Design review of the part built by this model. Coordinates are the model's own, in mm. A direction names the side the tool comes from. Round coordinates to 2 decimals unless told otherwise and drop trailing zeros. Write each loop counter-clockwise with the first axis right and the second up, starting at its lowest first coordinate (ties: lowest second). Pieces come first, ordered by that corner, then holes. Notation, with made-up numbers: (-4.75, -14) -> (46.25, -14) arc R22 ccw to (46.25, -2) -> close; hole circle Ø10 at (56, 24.5). An arc over 180 degrees is marked (long way). One line per question, with ' | ' between items. Start each with the question number.
1) Mouldability with a two-part tool opening along Z and no side actions: class faces 1 (the cylindrical face through (-85.51, 20.27, 4.03)), 2 (the cylindrical face through (-13.046, 7.296, 5.042)), 3 (the flat face through (-23, 4, 6)), 4 (the flat face through (-46, 79, 2)) as +Z half, -Z half, draft (parallel to the pull), parting line (faces both ways), or undercut.
2) For faces 5 (the flat face through (-6, 23, 5)), 6 (the flat face through (-67, 152, 6)), 7 (the cylindrical face through (-4.296, 10.389, 5.042)), 8 (the cylindrical face through (-8.31, 12.01, 5.04)), 9 (the flat face through (-85, 137, 6)), list the 3-axis set-ups (+Z, -Z, +X, -X, +Y, -Y) from which the entire face can be reached by the end or side of a thin tool; tool diameter is ignored.
3) Insertion check: pin 1 Ø1 at (y, z) = (19.5, 4.5) entering from +X; pin 2 Ø3 at (x, z) = (-35.5, 5.5) entering from -Y; pin 3 Ø10 at (x, y) = (-13.5, 95.5) entering from +Z. Each pin has a flat end and moves straight along its axis. Give the tip position at first contact, or say it passes through.
4) For probe 1 along Y at (x, z) = (-43, 6); probe 2 along X at (y, z) = (3.6, 5); probe 3 along Z at (x, y) = (-67, 151.3), list the stretches that pass through material, from the lowest coordinate up.
5) Consider section A-A (x = -39.5). Give the boundary of the cut face in (y, z), then the cut area to 3 significant figures.
6) Consider section B-B (y = 102.5). Give the boundary of the cut face in (x, z).
```python
from build123d import *

# Parameters (mm, degrees)
SKETCH_1_W                = 90
SKETCH_1_H                = 156
EXTRUDE_1_DEPTH           = 2
CHAMFER_1_SIZE            = 10
FILLET_648_R              = 2
EXTRUDE_2_DEPTH           = 6
SHELL_3_T                 = -4
SHELL_3_THICKNESS_2_DEPTH = 2
SKETCH_17_W               = 18.399609766
SKETCH_17_H               = 163.649147631
SKETCH_17_W_2             = 16.459731854
SKETCH_17_H_2             = 168.058563627
CUT_EXTRUDE_14_DEPTH      = 6
SKETCH_8_W                = 109.527726605
SKETCH_8_H                = 110
CUT_EXTRUDE_4177_DEPTH    = 6
EXTRUDE_5_DEPTH           = 6
SKETCH_5_R                = 0.8
CUT_EXTRUDE_5486_DEPTH    = 200
FILLET_5638_R             = 4
SKETCH_4_R                = 0.8
CUT_EXTRUDE_6124_DEPTH    = 100
SKETCH_6_W                = 5
SKETCH_6_H                = 14
EXTRUDE_C_DEPTH           = 6
SKETCH_9_R                = 0.8
CUT_EXTRUDE_C_DEPTH       = 50
SKETCH_23_R               = 1.6
CUT_EXTRUDE_16_DEPTH      = 1
CUT_EXTRUDE_START         = -1
SKETCH_24_R               = 1.6
CUT_EXTRUDE_17_DEPTH      = 1
SKETCH_22_R               = 1.6
CUT_EXTRUDE_15_DEPTH      = 1
SKETCH_13_R               = 1.6
CUT_EXTRUDE_10_DEPTH      = 1
SKETCH_18_W               = 2
SKETCH_18_H               = 96
EXTRUDE_4_DEPTH           = 6
FILLET_1_R                = 4
FILLET_2_R                = 0.5
SKETCH_25_W               = 24.531639896
SKETCH_25_H               = 27.877987264
CUT_EXTRUDE_18_DEPTH      = 10


with BuildPart() as part:
    # 草图1 → 凸台-拉伸1 (new body)
    with BuildSketch(Plane.XY):
        with Locations((-45, 78)):
            Rectangle(SKETCH_1_W, SKETCH_1_H)
    extrude(amount=EXTRUDE_1_DEPTH)

    # 倒角1
    chamfer_1_edges = [part.edges().sort_by_distance(p)[0] for p in [
        (0, 0, 1),
        (-90, 0, 1),
        (-90, 156, 1),
        (0, 156, 1),
    ]]
    chamfer(chamfer_1_edges, length=CHAMFER_1_SIZE)

    # Fillet 648
    fillet_648_edges = [part.edges().sort_by_distance(p)[0] for p in [
        (0, 146, 1),
        (0, 10, 1),
        (-80, 0, 1),
        (-10, 0, 1),
        (-90, 146, 1),
        (-90, 10, 1),
        (-10, 156, 1),
        (-80, 156, 1),
    ]]
    fillet(fillet_648_edges, radius=FILLET_648_R)

    # 草图2 → 凸台-拉伸2 (add)
    with BuildSketch(Plane.XY.offset(2)):
        Polygon((-78.757359313, 153), (-11.242640687, 153), (-3, 144.757359313), (-3, 11.242640687), (-11.242640687, 3), (-78.757359313, 3), (-87, 11.242640687), (-87, 144.757359313), align=None)
    extrude(amount=EXTRUDE_2_DEPTH)

    # 抽壳3
    shell_3_openings = [part.faces().sort_by_distance(p)[0] for p in [
        (-45, 78, 8),
    ]]
    offset(amount=SHELL_3_T, openings=shell_3_openings, kind=Kind.INTERSECTION)

    # 抽壳3 thickness 2 face (on inner face of the shell) → 抽壳3 thickness 2 (cut)
    with BuildSketch(Plane(origin=(-45, 78, 4), x_dir=(-1, 0, 0), z_dir=(0, 0, -1))):
        Polygon((38, -65.100505063), (32.100505063, -71), (-32.100505063, -71), (-38, -65.100505063), (-38, 65.100505063), (-32.100505063, 71), (32.100505063, 71), (38, 65.100505063), align=None)
    extrude(amount=SHELL_3_THICKNESS_2_DEPTH, mode=Mode.SUBTRACT)

    # 草图17 → 切除-拉伸14 (cut)
    with BuildSketch(Plane.XY.offset(8)):
        with Locations((-95.199804883, 77.855305794)):
            Rectangle(SKETCH_17_W, SKETCH_17_H)
        with Locations((4.229865927, 75.650597796)):
            Rectangle(SKETCH_17_W_2, SKETCH_17_H_2)
    extrude(amount=-CUT_EXTRUDE_14_DEPTH, mode=Mode.SUBTRACT)

    # 草图8 → Cut-Extrude 4177 (cut)
    with BuildSketch(Plane.XY.offset(8)):
        with Locations((-46.223461864, 78)):
            Rectangle(SKETCH_8_W, SKETCH_8_H)
    extrude(amount=-CUT_EXTRUDE_4177_DEPTH, mode=Mode.SUBTRACT)

    # 草图21 → 凸台-拉伸5 (add)
    with BuildSketch(Plane.XY.offset(2)):
        Polygon((-82, 142.100505063), (-82, 144.100505063), (-83, 143.100505063), (-83, 133), (-82, 133), align=None)
        Polygon((-8, 142.100505063), (-8, 144.100505063), (-7, 143.100505063), (-7, 133), (-8, 133), align=None)
        Polygon((-82, 13.899494937), (-82, 11.899494937), (-83, 12.899494937), (-83, 23), (-82, 23), align=None)
        Polygon((-8, 13.899494937), (-8, 11.899494937), (-7, 12.899494937), (-7, 23), (-8, 23), align=None)
    extrude(amount=EXTRUDE_5_DEPTH)

    # 草图5 → Cut-Extrude 5486 (cut)
    with BuildSketch(Plane(origin=(0, 3, 0), x_dir=(-1, 0, 0), z_dir=(0, -1, 0))):
        with Locations(Location((67, -5, 0), (0, 0, 90))):
            Circle(SKETCH_5_R)
        with Locations(Location((23, -5, 0), (0, 0, 90))):
            Circle(SKETCH_5_R)
        with Locations(Location((45, -5, 0), (0, 0, 90))):
            Circle(SKETCH_5_R)
    extrude(amount=-CUT_EXTRUDE_5486_DEPTH, mode=Mode.SUBTRACT)

    # Fillet 5638
    fillet_5638_edges = [part.edges().sort_by_distance(p)[0] for p in [
        (-4, 145.757359313, 5),
        (-86, 10.242640687, 5),
        (-86, 145.757359313, 5),
        (-4, 10.242640687, 5),
        (-78.757359313, 153, 5),
        (-78.757359313, 3, 5),
        (-11.242640687, 3, 5),
        (-11.242640687, 153, 5),
    ]]
    fillet(fillet_5638_edges, radius=FILLET_5638_R)

    # 草图4 → Cut-Extrude 6124 (cut)
    with BuildSketch(Plane.ZY.offset(87)):
        with Locations(Location((5, 137, 0), (0, 0, 270))):
            Circle(SKETCH_4_R)
        with Locations(Location((5, 19, 0), (0, 0, 270))):
            Circle(SKETCH_4_R)
    extrude(amount=-CUT_EXTRUDE_6124_DEPTH, mode=Mode.SUBTRACT)

    # 草图6 → C板固定 (add)
    with BuildSketch(Plane.XY.offset(2)):
        with Locations((-48.5, 134)):
            Rectangle(SKETCH_6_W, SKETCH_6_H)
        with Locations((-43.5, 22)):
            Rectangle(SKETCH_6_W, SKETCH_6_H)
    extrude(amount=EXTRUDE_C_DEPTH)

    # 草图9 → C板螺纹 (cut)
    with BuildSketch(Plane(origin=(-41, 0, 0), x_dir=(0, 0, -1), z_dir=(1, 0, 0))):
        with Locations(Location((-5, 26, 0), (0, 0, 90))):
            Circle(SKETCH_9_R)
        with Locations((-5, 130)):
            Circle(SKETCH_9_R)
    extrude(amount=-CUT_EXTRUDE_C_DEPTH, mode=Mode.SUBTRACT)

    # 草图23 → 切除-拉伸16 (cut)
    with BuildSketch(Plane.ZY.offset(86)):
        with Locations(Location((5, 137, 0), (0, 0, 270))):
            Circle(SKETCH_23_R)
        with Locations(Location((5, 19, 0), (0, 0, 270))):
            Circle(SKETCH_23_R)
    extrude(amount=-CUT_EXTRUDE_16_DEPTH, mode=Mode.SUBTRACT)

    # 草图24 → 切除-拉伸17 (cut)
    with BuildSketch(Plane(origin=(-4, 0, 0), x_dir=(0, 0, -1), z_dir=(1, 0, 0)).offset(CUT_EXTRUDE_START)):
        with Locations(Location((-5, 19, 0), (0, 0, 270))):
            Circle(SKETCH_24_R)
        with Locations(Location((-5, 137, 0), (0, 0, 270))):
            Circle(SKETCH_24_R)
    extrude(amount=CUT_EXTRUDE_17_DEPTH, mode=Mode.SUBTRACT)

    # 草图22 → 切除-拉伸15 (cut)
    with BuildSketch(Plane(origin=(0, 3, 0), x_dir=(-1, 0, 0), z_dir=(0, -1, 0))):
        with Locations(Location((67, -5, 0), (0, 0, 90))):
            Circle(SKETCH_22_R)
        with Locations(Location((45, -5, 0), (0, 0, 90))):
            Circle(SKETCH_22_R)
        with Locations(Location((23, -5, 0), (0, 0, 90))):
            Circle(SKETCH_22_R)
    extrude(amount=-CUT_EXTRUDE_15_DEPTH, mode=Mode.SUBTRACT)

    # 草图13 → 切除-拉伸10 (cut)
    with BuildSketch(Plane(origin=(0, 153, 0), x_dir=(1, 0, 0), z_dir=(0, 1, 0)).offset(CUT_EXTRUDE_START)):
        with Locations(Location((-67, -5, 0), (0, 0, 90))):
            Circle(SKETCH_13_R)
        with Locations(Location((-45, -5, 0), (0, 0, 90))):
            Circle(SKETCH_13_R)
        with Locations(Location((-23, -5, 0), (0, 0, 90))):
            Circle(SKETCH_13_R)
    extrude(amount=CUT_EXTRUDE_10_DEPTH, mode=Mode.SUBTRACT)

    # 草图18 → 凸台-拉伸4 (add)
    with BuildSketch(Plane.XY.offset(2)):
        with Locations((-87.078063163, 78)):
            Rectangle(SKETCH_18_W, SKETCH_18_H)
    extrude(amount=EXTRUDE_4_DEPTH)

    # 圆角1
    fillet_1_edges = [part.edges().sort_by_distance(p)[0] for p in [
        (-77.100505063, 149, 5),
        (-77.100505063, 7, 5),
        (-12.899494937, 7, 5),
        (-12.899494937, 149, 5),
        (-82, 144.100505063, 5),
        (-8, 144.100505063, 5),
        (-82, 11.899494937, 5),
        (-8, 11.899494937, 5),
    ]]
    fillet(fillet_1_edges, radius=FILLET_1_R)

    # 圆角2
    fillet_2_edges = [part.edges().sort_by_distance(p)[0] for p in [
        (-86, 133, 5),
        (-86, 23, 5),
        (-4, 23, 5),
        (-4, 133, 5),
        (-82, 133, 5),
        (-8, 133, 5),
        (-82, 23, 5),
        (-8, 23, 5),
        (-51, 141, 5),
        (-51, 127, 5),
        (-46, 127, 5),
        (-46, 141, 5),
        (-41, 15, 5),
        (-41, 29, 5),
        (-46, 29, 5),
        (-46, 15, 5),
        (-88.078063163, 126, 5),
        (-88.078063163, 30, 5),
        (-86.078063163, 30, 5),
        (-86.078063163, 126, 5),
    ]]
    fillet(fillet_2_edges, radius=FILLET_2_R)

    # 草图25 → 切除-拉伸18 (cut)
    with BuildSketch(Plane.XY.offset(2)):
        with Locations((-48.129545647, 132.25729865)):
            Rectangle(SKETCH_25_W, SKETCH_25_H)
    extrude(amount=CUT_EXTRUDE_18_DEPTH, mode=Mode.SUBTRACT)


solid = part.part
```
From the geometry:
1) face 1: undercut | face 2: draft | face 3: undercut | face 4: +Z half
2) face 5: +Z, +X | face 6: +Y | face 7: +Z, +X, -Y | face 8: +Z | face 9: -X
3) pin 1: stops at x = -5 | pin 2: stops at y = 3 | pin 3: stops at z = 2
4) probe 1: y = 3 to 7, 15 to 29, 149 to 153 | probe 2: x = -79.21 to -68.6, -65.4 to -46.6, -43.4 to -24.6, -21.4 to -10.79 | probe 3: z = 0 to 4.2, 5.8 to 8
5) outline: (0, 0) -> (156, 0) -> (156, 2) -> (153, 2) -> (153, 8) -> (149, 8) -> (149, 2) -> (7, 2) -> (7, 8) -> (3, 8) -> (3, 2) -> (0, 2) -> close | area: 360 mm2
6) outline: (-90, 0) -> (0, 0) -> (0, 2) -> (-86.08, 2) -> (-86.08, 8) -> (-88.08, 8) -> (-88.08, 2) -> (-90, 2) -> close
